from build123d import *

# Parameters (mm, degrees)
SKETCH1_W           = 80
SKETCH1_H           = 110
BOSS_EXTRUDE1_DEPTH = 5
SKETCH1_3_R         = 3.4
BOSS_EXTRUDE3_DEPTH = 15
BOSS_EXTRUDE4_DEPTH = 25
SKETCH2_W           = 80
SKETCH2_H           = 5
BOSS_EXTRUDE5_DEPTH = 60
SKETCH3_W           = 5
SKETCH3_H           = 38
BOSS_EXTRUDE6_DEPTH = 15
SKETCH4_W           = 5
SKETCH4_H           = 35
BOSS_EXTRUDE7_DEPTH = 90
FILLET1_R           = 10
CUT_EXTRUDE1_START  = -105
SKETCH5_W           = 2
SKETCH5_H           = 5.3
CUT_EXTRUDE1_DEPTH  = 105
CUT_EXTRUDE2_REACH  = 92.692
FILLET2_R           = 5


with BuildPart() as part:
    # Sketch1 → Boss-Extrude1 (new body)
    with BuildSketch(Plane.XY):
        Rectangle(SKETCH1_W, SKETCH1_H)
    extrude(amount=BOSS_EXTRUDE1_DEPTH)

    # Sketch1<3> → Boss-Extrude3 (add)
    with BuildSketch(Plane.XY):
        with Locations((-29, 9)):
            Circle(SKETCH1_3_R)
        with Locations((29, 9)):
            Circle(SKETCH1_3_R)
        with Locations((29, -40)):
            Circle(SKETCH1_3_R)
        with Locations((-29, -40)):
            Circle(SKETCH1_3_R)
    extrude(amount=BOSS_EXTRUDE3_DEPTH)

    # Sketch1<4> → Boss-Extrude4 (add)
    with BuildSketch(Plane.XY):
        with BuildLine():
            Line((-25.6, 15.65), (-29.15, 15.65))
            ThreePointArc((-29.15, 15.65), (-33.746194078, 13.746194078), (-35.65, 9.15))
            Line((-35.65, 9.15), (-35.65, 5.6))
            Line((-35.65, 5.6), (-32.65, 5.6))
            Line((-32.65, 5.6), (-32.65, 9.15))
            ThreePointArc((-32.65, 9.15), (-31.624873734, 11.624873734), (-29.15, 12.65))
            Line((-29.15, 12.65), (-25.6, 12.65))
            Line((-25.6, 12.65), (-25.6, 15.65))
        make_face()
        with BuildLine():
            Line((29.15, 15.65), (25.6, 15.65))
            Line((25.6, 15.65), (25.6, 12.65))
            Line((25.6, 12.65), (29.15, 12.65))
            ThreePointArc((29.15, 12.65), (31.624873734, 11.624873734), (32.65, 9.15))
            Line((32.65, 9.15), (32.65, 5.6))
            Line((32.65, 5.6), (35.65, 5.6))
            Line((35.65, 5.6), (35.65, 9.15))
            ThreePointArc((35.65, 9.15), (33.746194078, 13.746194078), (29.15, 15.65))
        make_face()
        with BuildLine():
            Line((35.65, -40.15), (35.65, -36.6))
            Line((35.65, -36.6), (32.65, -36.6))
            Line((32.65, -36.6), (32.65, -40.15))
            ThreePointArc((32.65, -40.15), (31.624873734, -42.624873734), (29.15, -43.65))
            Line((29.15, -43.65), (25.6, -43.65))
            Line((25.6, -43.65), (25.6, -46.65))
            Line((25.6, -46.65), (29.15, -46.65))
            ThreePointArc((29.15, -46.65), (33.746194078, -44.746194078), (35.65, -40.15))
        make_face()
        with BuildLine():
            Line((-32.65, -36.6), (-35.65, -36.6))
            Line((-35.65, -36.6), (-35.65, -40.15))
            ThreePointArc((-35.65, -40.15), (-33.746194078, -44.746194078), (-29.15, -46.65))
            Line((-29.15, -46.65), (-25.6, -46.65))
            Line((-25.6, -46.65), (-25.6, -43.65))
            Line((-25.6, -43.65), (-29.15, -43.65))
            ThreePointArc((-29.15, -43.65), (-31.624873734, -42.624873734), (-32.65, -40.15))
            Line((-32.65, -40.15), (-32.65, -36.6))
        make_face()
    extrude(amount=BOSS_EXTRUDE4_DEPTH)

    # Sketch2 → Boss-Extrude5 (add)
    with BuildSketch(Plane.XY.offset(5)):
        with Locations((0, -52.5)):
            Rectangle(SKETCH2_W, SKETCH2_H)
    extrude(amount=BOSS_EXTRUDE5_DEPTH)

    # Sketch3 → Boss-Extrude6 (add)
    with BuildSketch(Plane(origin=(0, -50, 0), x_dir=(1, 0, 0), z_dir=(0, 1, 0))):
        with Locations((-37.5, -46)):
            Rectangle(SKETCH3_W, SKETCH3_H)
        with Locations((37.5, -46)):
            Rectangle(SKETCH3_W, SKETCH3_H)
    extrude(amount=BOSS_EXTRUDE6_DEPTH)

    # Sketch4 → Boss-Extrude7 (add)
    with BuildSketch(Plane(origin=(0, -35, 0), x_dir=(1, 0, 0), z_dir=(0, 1, 0))):
        with Locations((-37.5, -47.5)):
            Rectangle(SKETCH4_W, SKETCH4_H)
        with Locations((37.5, -47.5)):
            Rectangle(SKETCH4_W, SKETCH4_H)
    extrude(amount=BOSS_EXTRUDE7_DEPTH)

    # Fillet1
    # the kernel refuses this fillet: 10 mm, written as the material it adds along each edge
    with BuildSketch(Plane(origin=(-35, -50, 65), x_dir=(1, 0, 0), z_dir=(0, 0, -1)), Plane(origin=(35, -50, 27), x_dir=(-1, 0, 0), z_dir=(0, 0, 1))) as fillet1_piece_1:
        with BuildLine():
            CenterArc((FILLET1_R, -FILLET1_R), FILLET1_R, 90, 90)
            Line((0, -FILLET1_R), (0, 0))
            Line((0, 0), (FILLET1_R, 0))
        make_face()
    extrude(amount=38)
    with BuildSketch(Plane(origin=(40, -50, 5), x_dir=(0, 1, 0), z_dir=(-1, 0, 0))) as fillet1_piece_2:
        with BuildLine():
            CenterArc((FILLET1_R, -FILLET1_R), FILLET1_R, 90, 90)
            Line((0, -FILLET1_R), (0, 0))
            Line((0, 0), (FILLET1_R, 0))
        make_face()
    extrude(amount=80)

    # Sketch5 → Cut-Extrude1 (cut)
    with BuildSketch(Plane(origin=(0, 55, 0), x_dir=(1, 0, 0), z_dir=(0, 1, 0)).offset(CUT_EXTRUDE1_START)):
        with Locations((-36, -54.275)):
            Rectangle(SKETCH5_W, SKETCH5_H)
        with Locations((36, -54.275)):
            Rectangle(SKETCH5_W, SKETCH5_H)
    extrude(amount=CUT_EXTRUDE1_DEPTH, mode=Mode.SUBTRACT)

    # Sketch6 → Cut-Extrude2 (cut, up to next)
    with BuildSketch(Plane.XY.offset(5), mode=Mode.PRIVATE) as cut_extrude2_sk1:
        Polygon((0, 45.659569378), (25.6, 15.65), (-25.6, 15.65), align=None)
    cut_extrude2_tool1 = extrude(cut_extrude2_sk1.sketch, amount=-CUT_EXTRUDE2_REACH, mode=Mode.PRIVATE) & part.part
    # Sketch6 → Cut-Extrude2 (cut, up to next)
    with BuildSketch(Plane.XY.offset(5), mode=Mode.PRIVATE) as cut_extrude2_sk2:
        Polygon((-25.6, 15.65), (0, -6.188367347), (25.6, 15.65), align=None)
    cut_extrude2_tool2 = extrude(cut_extrude2_sk2.sketch, amount=-CUT_EXTRUDE2_REACH, mode=Mode.PRIVATE) & part.part
    # Sketch6 → Cut-Extrude2 (cut, up to next)
    with BuildSketch(Plane.XY.offset(5), mode=Mode.PRIVATE) as cut_extrude2_sk3:
        Polygon((-35.65, -36.6), (-10.915550239, -15.5), (-35.65, 5.6), align=None)
    cut_extrude2_tool3 = extrude(cut_extrude2_sk3.sketch, amount=-CUT_EXTRUDE2_REACH, mode=Mode.PRIVATE) & part.part
    # Sketch6 → Cut-Extrude2 (cut, up to next)
    with BuildSketch(Plane.XY.offset(5), mode=Mode.PRIVATE) as cut_extrude2_sk4:
        Polygon((-17.804545455, -40), (17.804545455, -40), (0, -24.811632653), align=None)
    cut_extrude2_tool4 = extrude(cut_extrude2_sk4.sketch, amount=-CUT_EXTRUDE2_REACH, mode=Mode.PRIVATE) & part.part
    # Sketch6 → Cut-Extrude2 (cut, up to next)
    with BuildSketch(Plane.XY.offset(5), mode=Mode.PRIVATE) as cut_extrude2_sk5:
        Polygon((10.915550239, -15.5), (35.65, -36.6), (35.65, 5.6), align=None)
    cut_extrude2_tool5 = extrude(cut_extrude2_sk5.sketch, amount=-CUT_EXTRUDE2_REACH, mode=Mode.PRIVATE) & part.part
    add(cut_extrude2_tool1.solids().sort_by_distance((0, 25.65319, 5))[0], mode=Mode.SUBTRACT)
    add(cut_extrude2_tool2.solids().sort_by_distance((0, 8.370544, 5))[0], mode=Mode.SUBTRACT)
    add(cut_extrude2_tool3.solids().sort_by_distance((-27.405183, -15.5, 5))[0], mode=Mode.SUBTRACT)
    add(cut_extrude2_tool4.solids().sort_by_distance((0, -34.937211, 5))[0], mode=Mode.SUBTRACT)
    add(cut_extrude2_tool5.solids().sort_by_distance((27.405183, -15.5, 5))[0], mode=Mode.SUBTRACT)

    # Fillet2
    # the kernel refuses this fillet: 5 mm, written as the material it adds along each edge
    with BuildSketch(Plane(origin=(17.804545455, -40, 5), x_dir=(-1, 0, 0), z_dir=(0, 0, -1))) as fillet2_piece_1:
        with BuildLine():
            CenterArc((FILLET2_R * 2.71308210373, FILLET2_R), FILLET2_R, 130.466208854, 139.533791146)
            Line((FILLET2_R * 2.06408263048, FILLET2_R * 1.7607888562), (0, 0))
            Line((0, 0), (FILLET2_R * 2.71308210373, 0))
        make_face()
    extrude(amount=5)
    with BuildSketch(Plane(origin=(0, -24.811632653, 5), x_dir=(0.7607888562020934, -0.6489994732499483, 0), z_dir=(0, 0, -1)), Plane(origin=(0, -6.188367347, 5), x_dir=(-0.7607888562020926, 0.6489994732499494, 0), z_dir=(0, 0, -1))) as fillet2_piece_2:
        with BuildLine():
            CenterArc((FILLET2_R * 0.85306122449, FILLET2_R), FILLET2_R, 189.067582292, 80.932417708)
            Line((-FILLET2_R * 0.134441909369, FILLET2_R * 0.842400632557), (0, 0))
            Line((0, 0), (FILLET2_R * 0.85306122449, 0))
        make_face()
    extrude(amount=5)
    with BuildSketch(Plane(origin=(-17.804545455, -40, 5), x_dir=(1, 0, 0), z_dir=(0, 0, -1))) as fillet2_piece_3:
        with BuildLine():
            CenterArc((FILLET2_R * 2.71308210373, -FILLET2_R), FILLET2_R, 90, 139.533791146)
            Line((FILLET2_R * 2.06408263048, -FILLET2_R * 1.7607888562), (0, 0))
            Line((0, 0), (FILLET2_R * 2.71308210373, 0))
        make_face()
    extrude(amount=5)
    with BuildSketch(Plane(origin=(-35.65, 5.6, 5), x_dir=(0, -1, 0), z_dir=(0, 0, -1)), Plane(origin=(35.65, -36.6, 5), x_dir=(0, 1, 0), z_dir=(0, 0, -1))) as fillet2_piece_4:
        with BuildLine():
            CenterArc((FILLET2_R * 2.16748636604, -FILLET2_R), FILLET2_R, 90, 130.466208854)
            Line((FILLET2_R * 1.40669750983, -FILLET2_R * 1.64899947325), (0, 0))
            Line((0, 0), (FILLET2_R * 2.16748636604, 0))
        make_face()
    extrude(amount=5)
    with BuildSketch(Plane(origin=(-10.915550239, -15.5, 5), x_dir=(-0.7607888562020928, -0.6489994732499492, 0), z_dir=(0, 0, -1)), Plane(origin=(10.915550239, -15.5, 5), x_dir=(0.760788856202093, 0.648999473249949, 0), z_dir=(0, 0, -1)), Plane(origin=(0, 45.659569378, 5), x_dir=(0.6489994732499487, -0.7607888562020931, 0), z_dir=(0, 0, -1))) as fillet2_piece_5:
        with BuildLine():
            CenterArc((FILLET2_R * 1.17224880383, FILLET2_R), FILLET2_R, 170.932417708, 99.067582292)
            Line((FILLET2_R * 0.184745669969, FILLET2_R * 1.15759936744), (0, 0))
            Line((0, 0), (FILLET2_R * 1.17224880383, 0))
        make_face()
    extrude(amount=5)
    with BuildSketch(Plane(origin=(-35.65, -36.6, 5), x_dir=(0, 1, 0), z_dir=(0, 0, -1)), Plane(origin=(35.65, 5.6, 5), x_dir=(0, -1, 0), z_dir=(0, 0, -1))) as fillet2_piece_6:
        with BuildLine():
            CenterArc((FILLET2_R * 2.16748636604, FILLET2_R), FILLET2_R, 139.533791146, 130.466208854)
            Line((FILLET2_R * 1.40669750983, FILLET2_R * 1.64899947325), (0, 0))
            Line((0, 0), (FILLET2_R * 2.16748636604, 0))
        make_face()
    extrude(amount=5)
    with BuildSketch(Plane(origin=(25.6, 15.65, 5), x_dir=(-0.6489994732499493, 0.7607888562020927, 0), z_dir=(0, 0, -1))) as fillet2_piece_7:
        with BuildLine():
            CenterArc((FILLET2_R, -FILLET2_R), FILLET2_R, 90, 90)
            Line((0, -FILLET2_R), (0, 0))
            Line((0, 0), (FILLET2_R, 0))
        make_face()
    extrude(amount=5)
    with BuildSketch(Plane(origin=(-25.6, 15.65, 5), x_dir=(0.648999473249949, 0.7607888562020928, 0), z_dir=(0, 0, -1))) as fillet2_piece_8:
        with BuildLine():
            CenterArc((FILLET2_R, FILLET2_R), FILLET2_R, 180, 90)
            Line((0, FILLET2_R), (0, 0))
            Line((0, 0), (FILLET2_R, 0))
        make_face()
    extrude(amount=5)


solid = part.part
The listing builds one solid part. Answer for the finished solid, in the listing's coordinates (mm). A direction names the side the tool comes from. Coordinates: 2 decimals unless noted, no trailing zeros. Order: outer loops, then holes, each group sorted by start corner. A loop starts at its lowest first (then second) coordinate and runs counter-clockwise, first axis right, second up.
Q1. A cutting plane is placed at B-B, the plane y = 33. Write down the section's boundary in (x, z) (3 decimals), and give its area (3 significant figures).
Q2. A cutting plane is placed at D-D, the plane y = -17.5. Write down the section's boundary in (x, z) (3 decimals).
Q3. A cutting plane is placed at A-A, the plane x = 11.5. Write down the section's boundary in (y, z), and give its area (3 significant figures).
Q4. For a pull along Y with two mould halves and no side action, classify faces 1 (the face through (29, -40, 15)), 2 (the face through (-1, 55, 2)), 3 (the face through (0.049, -4.616, 2.535)), 4 (the face through (35, 7, 61)) as pulls with the +Y half, pulls with the -Y half, needs draft (parallel to the pull), parting line crosses it, or undercut.
Q5. Consider line 1 (Y direction, x = -29, z = 23); line 2 (X direction, y = 21.5, z = 42.5); line 3 (Y direction, x = 28.5, z = 13). Determine where each line is inside the solid, lowest interval first.
Q6. A cutting plane is placed at C-C, the plane z = 22.5. State how many separate pieces and enclosed holes the cut face has, and give its area (3 significant figures).
Q7. Which of the six approach directions +Z, -Z, +X, -X, +Y, -Y give full straight-line access (tool end or side, diameter ignored) to faces 5 (the face through (-35, -45, 54)), 6 (the face through (-0.061, 42.955, 2.535)), 7 (the face through (30.828, -37.133, 9.93)), 8 (the face through (-36, -44, 27))?
Q8. Given P1, Ø4, axis at y = -38.5, z = 11, coming from the -X side; P2, Ø10, axis at x = -24, z = 57, coming from the +Y side; P3, Ø6, axis at x = -14, y = -42, coming from the +Z side; P4, Ø2, axis at x = 8.5, y = 3, coming from the +Z side, each flat-ended and moving along its own axis, determine where each tip first touches the part or whether it passes through.
Answers follow:
1. outline: (-40, 0) - (-10.799, 0) - (-10.799, 5) - (-40, 5) - close; (-40, 30) - (-35, 30) - (-35, 51.625) - (-37, 51.625) - (-37, 56.925) - (-35, 56.925) - (-35, 65) - (-40, 65) - close; (10.799, 0) - (40, 0) - (40, 5) - (10.799, 5) - close; (35, 30) - (40, 30) - (40, 65) - (35, 65) - (35, 56.925) - (37, 56.925) - (37, 51.625) - (35, 51.625) - close
1. area: 621 mm2
2. outline: (-40, 0) - (-35.65, 0) - (-35.65, 5) - (-40, 5) - close; (-40, 30) - (-35, 30) - (-35, 51.625) - (-37, 51.625) - (-37, 56.925) - (-35, 56.925) - (-35, 65) - (-40, 65) - close; (-14.037, 0) - (14.037, 0) - (14.037, 5) - (-14.037, 5) - close; (35, 30) - (40, 30) - (40, 65) - (35, 65) - (35, 56.925) - (37, 56.925) - (37, 51.625) - (35, 51.625) - close; (35.65, 0) - (40, 0) - (40, 5) - (35.65, 5) - close
3. outline: (-55, 0) - (3.62, 0) - (3.62, 5) - (-40, 5) arc R10 cw to (-50, 15) - (-50, 65) - (-55, 65) - close; (32.18, 0) - (55, 0) - (55, 5) - (32.18, 5) - close
3. area: 729 mm2
4. face 1: undercut
4. face 2: pulls with the +Y half
4. face 3: undercut
4. face 4: needs draft
5. line 1: y = -55 to -50, -46.65 to -43.65, 12.65 to 15.65
5. line 2: x = -40 to -35, 35 to 40
5. line 3: y = -55 to -49.8, -46.65 to -43.65, -43.36 to -36.64, 5.64 to 12.36, 12.65 to 15.65
6. separate pieces: 5
6. enclosed holes: 0
6. area: 579 mm2
7. face 5: +Y
7. face 6: +Z, -Z
7. face 7: +Z
7. face 8: +X, -X, +Y
8. P1: stops at x = -35.65
8. P2: stops at y = -49.17
8. P3: stops at z = 6.34
8. P4: passes through
